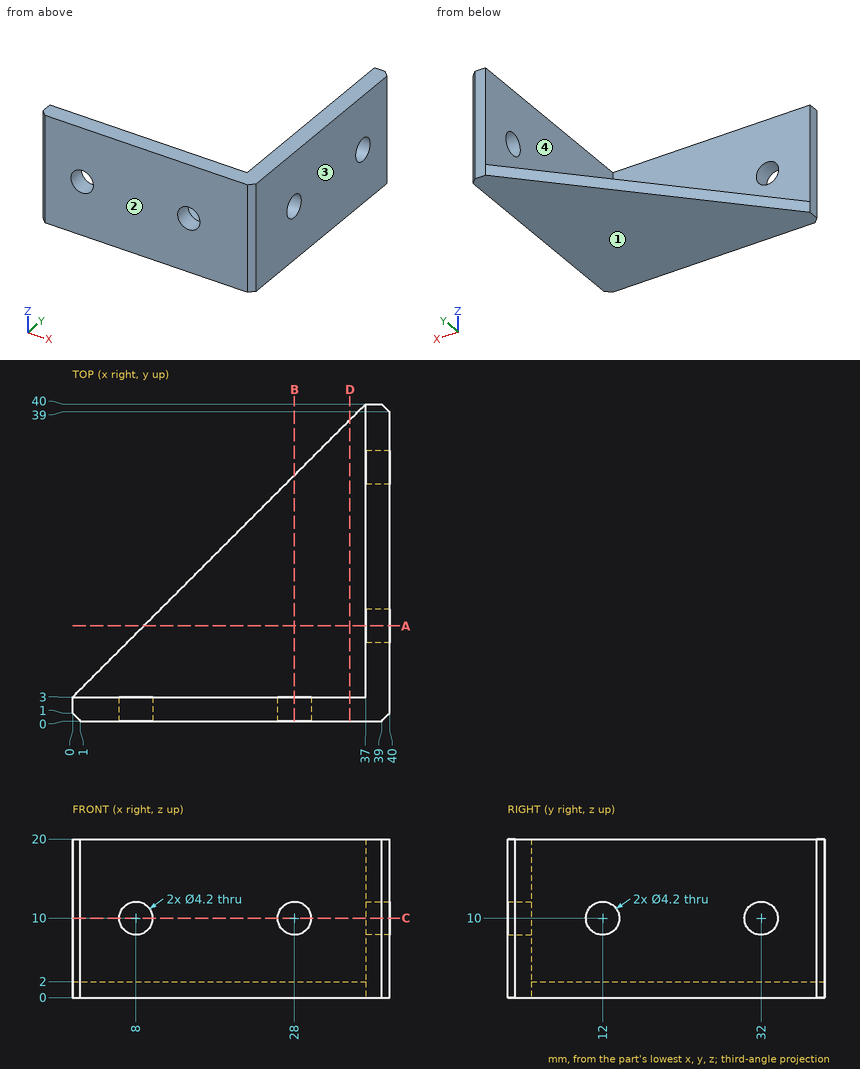
Study the drawing (mm; zero at the part's minimum x, y, z) and answer. A direction names the side the tool comes from. Give positions to 0.01 mm unless a question says otherwise; leave off trailing zeros. Write each loop counter-clockwise with the first axis right and the second up, starting at its lowest first coordinate (ties: lowest second). Pieces come first, ordered by that corner, then holes. Notation, with made-up numbers: (-5, 85) - (51, 85) arc R18 ccw to (51, 103) - close; hole circle Ø4 at (22.25, 63.5). An arc over 180 degrees is marked (long way). One line per question, with ' | ' between items. Start each with the question number.
1. Section D-D, the plane x = 35 is taken. Determine the outline of the cut face in (y, z), then the cut area to 3 significant figures.
2. Given P1, Ø4, axis at x = 8.5, z = 6.5, coming from the +Y side; P2, Ø3, axis at x = 27.5, z = 2.5, coming from the +Y side; P3, Ø5, axis at y = 32, z = 10, coming from the +X side, each flat-ended and moving along its own axis, determine where each tip first touches the part or whether it passes through.
3. For the marked faces 3 and 4, determine the directions among +Z, -Z, +X, -X, +Y, -Y from which every point of the face is accessible in a straight line to the end or side of a thin tool.
4. Section A-A, the plane y = 12 is taken. Determine the outline of the cut face in (x, z).
5. Section B-B, the plane x = 28 is taken. Determine the outline of the cut face in (y, z), then the cut area to 3 significant figures.
6. Section C-C, the plane z = 10 is taken. Determine the outline of the cut face in (x, y).
7. Determine the mould class of the marked faces 1 and 2 for opening direction Z: +Z half, -Z half, draft (parallel to the pull), parting line (faces both ways), or undercut.
8. Straight lines are drawn through the part: line 1 (X direction, y = 2.1, z = 10); line 2 (X direction, y = 12.5, z = 14); line 3 (Y direction, x = 16.5, z = 6.5). For each, find the intervals that lie inside material, in ascending order.
Result:
1) outline: (0, 0) - (38, 0) - (38, 2) - (3, 2) - (3, 20) - (0, 20) - close | area: 130 mm2
2) P1: stops at y = 3 | P2: stops at y = 31.91 | P3: stops at x = 40
3) face 3: +Z, -Z, +X, +Y, -Y | face 4: +Z, -X, +Y
4) outline: (9, 0) - (40, 0) - (40, 7.9) - (37, 7.9) - (37, 2) - (9, 2) - close; (37, 12.1) - (40, 12.1) - (40, 20) - (37, 20) - close
5) outline: (0, 0) - (31, 0) - (31, 2) - (3, 2) - (3, 7.9) - (0, 7.9) - close; (0, 12.1) - (3, 12.1) - (3, 20) - (0, 20) - close | area: 103 mm2
6) outline: (0, 1) - (1, 0) - (5.9, 0) - (5.9, 3) - (0, 3) - close; (10.1, 0) - (25.9, 0) - (25.9, 3) - (10.1, 3) - close; (30.1, 0) - (39, 0) - (40, 1) - (40, 9.9) - (37, 9.9) - (37, 3) - (30.1, 3) - close; (37, 14.1) - (40, 14.1) - (40, 29.9) - (37, 29.9) - close; (37, 34.1) - (40, 34.1) - (40, 39) - (39, 40) - (37, 40) - close
7) face 1: -Z half | face 2: draft
8) line 1: x = 0 to 5.9, 10.1 to 25.9, 30.1 to 40 | line 2: x = 37 to 40 | line 3: y = 0 to 3
